Design review of the part built by this model. Coordinates are the model's own, in mm. Round coordinates to 2 decimals unless told otherwise and drop trailing zeros. Write each loop counter-clockwise with the first axis right and the second up, starting at its lowest first coordinate (ties: lowest second). Pieces come first, ordered by that corner, then holes. Notation, with made-up numbers: (80, -20) -> (97, -20) arc R18 ccw to (97, -16) -> close; hole circle Ø11 at (40, 59). An arc over 180 degrees is marked (long way). One line per question, with ' | ' between items. Start each with the question number.
1) Mouldability with a two-part tool opening along X and no side actions: class faces 1 (the cylindrical face through (26.965, 357.707, 1.972)), 2 (the cylindrical face through (-15.304, 340.441, 1.972)), 3 (the flat face through (29, 156, 4)) as +X half, -X half, draft (parallel to the pull), parting line (faces both ways), or undercut.
2) For probe 1 along X at (y, z) = (242, 1.2); probe 2 along X at (y, z) = (-17, 2.6); probe 3 along Y at (x, z) = (6.5, 2.8), list the stretches that pass through material, from the lowest coordinate up.
3) Consider section A-A (y = 93.5). Give the boundary of the cut face in (x, z), then the cut area to 3 significant figures.
4) Insertion check: pin 1 Ø2 at (x, z) = (19.5, 3.5) entering from +Y. The pin has a flat end and moves straight along its axis. Give the tip position at first contact, or say it passes through.
5) Consider section C-C (y = -16). Give the boundary of the cut face in (x, z), then the cut area to 3 significant figures.
6) Consider section D-D (y = 40). Give the boundary of the cut face in (x, z), then the cut area to 3 significant figures.
```python
from build123d import *

# Parameters (mm, degrees)
F1_DEPTH = 4
F2_R     = 25.39999


# Not quite as in the source:
# - a fillet or chamfer is up to 0.001 mm smaller than in the source, because OpenCascade refuses the exact size


with BuildPart() as f1:
    # F0 (on Top) → F1 (new body)
    with BuildSketch(Plane.XY):
        with BuildLine():
            Line((25.4, 88.9), (25.4, 27.783106151))
            ThreePointArc((25.4, 27.783106151), (39.0875817391, 57.0211124393), (44.1814440725, 88.9))
            Line((44.1814440725, 88.9), (44.1814440725, 317.5))
            ThreePointArc((44.1814440725, 317.5), (26.6541395651, 358.2459104505), (0, 393.7))
            ThreePointArc((0, 393.7), (-26.9370466698, 358.2864987651), (-44.7185559275, 317.5))
            Line((-44.7185559275, 317.5), (-44.7185559275, 88.9))
            ThreePointArc((-44.7185559275, 88.9), (-39.2808523641, 57.0071475451), (-25.4, 27.783106151))
            Line((-25.4, 27.783106151), (-25.4, 81.8970223493))
            ThreePointArc((-25.4, 81.8970223493), (-25.7287156311, 85.5486031353), (-25.9225594861, 89.209821616))
            Line((-25.9225594861, 89.209821616), (-25.9225594861, 314.6655596019))
            ThreePointArc((-25.9225594861, 314.6655596019), (-15.1225925717, 340.7930484479), (-0.0869368678, 364.7349367673))
            ThreePointArc((-0.0869368678, 364.7349367673), (14.7574318658, 340.7960081036), (25.385447631, 314.7101331987))
            Line((25.385447631, 314.7101331987), (25.385447631, 89.0840377413))
            ThreePointArc((25.385447631, 89.0840377413), (25.3835184902, 88.992017936), (25.3815021522, 88.9))
            Line((25.3815021522, 88.9), (25.4, 88.9))
        make_face()
        with BuildLine():
            Line((-25.4, -88.9), (25.4, -88.9))
            Line((25.4, -88.9), (25.4, 27.783106151))
            ThreePointArc((25.4, 27.783106151), (13.8352633227, 12.8536673819), (0, 0))
            ThreePointArc((0, 0), (-13.8130547318, 12.8739710228), (-25.4, 27.783106151))
            Line((-25.4, 27.783106151), (-25.4, -88.9))
        make_face()
        with BuildLine():
            ThreePointArc((0, 0), (13.8352633227, 12.8536673819), (25.4, 27.783106151))
            Line((25.4, 27.783106151), (25.4, 88.9))
            Line((25.4, 88.9), (25.3815021522, 88.9))
            ThreePointArc((25.3815021522, 88.9), (18.4387554256, 54.950742752), (0.0203713554, 25.5991341412))
            ThreePointArc((0.0203713554, 25.5991341412), (-17.1734173627, 51.7235821598), (-25.4, 81.8970223493))
            Line((-25.4, 81.8970223493), (-25.4, 27.783106151))
            ThreePointArc((-25.4, 27.783106151), (-13.8130547318, 12.8739710228), (0, 0))
        make_face()
    extrude(amount=F1_DEPTH)

    # F2 (radius 25.4 in the source; OpenCascade refuses exactly that, so slightly less here)
    f2_edges = [f1.edges().sort_by_distance(p)[0] for p in [
        (-25.4, -88.9, 2),
        (25.4, -88.9, 2),
    ]]
    fillet(f2_edges, radius=F2_R)


solid = f1.part
```
From the geometry:
1) face 1: +X half | face 2: undercut | face 3: draft
2) probe 1: x = -44.72 to -25.92, 25.39 to 44.18 | probe 2: x = -25.4 to 25.4 | probe 3: y = -88.05 to 33.5, 355.2 to 386.55
3) outline: (-44.72, 0) -> (-25.92, 0) -> (-25.92, 4) -> (-44.72, 4) -> close; (25.39, 0) -> (44.18, 0) -> (44.18, 4) -> (25.39, 4) -> close | area: 150 mm2
4) pin 1: stops at y = 371.07
5) outline: (-25.4, 0) -> (25.4, 0) -> (25.4, 4) -> (-25.4, 4) -> close | area: 203 mm2
6) outline: (-32.41, 0) -> (-10.9, 0) -> (-10.9, 4) -> (-32.41, 4) -> close; (10.89, 0) -> (32.34, 0) -> (32.34, 4) -> (10.89, 4) -> close | area: 172 mm2
